```python
from build123d import *

# Parameters (mm, degrees)
BASPROSKE_W         = 6
BASPROSKE_H         = 15
TOOTHCUT_DEPTH      = 23.045407685
TEETHCUTS_COUNT     = 18
TEETHCUTS_ANGLE     = 340
BORSKE_R            = 1.5
BORE_DEPTH          = 50.0000508
EXTRUDE_2_DEPTH     = 6
SKETCH_2_R          = 1.65
CUT_EXTRUDE_1_DEPTH = 6
SKETCH_3_R          = 10.25
CUT_EXTRUDE_2_DEPTH = 2


with BuildPart() as part:
    # BasProSke → Base-Revolve (revolve)
    with BuildSketch(Plane(origin=(0, 0, 0), x_dir=(1, 0, 0), z_dir=(0, 1, 0)), mode=Mode.PRIVATE) as base_revolve_sk:
        with Locations((3, 7.5)):
            Rectangle(BASPROSKE_W, BASPROSKE_H)
    revolve(base_revolve_sk.sketch.rotate(Axis((-10, 0, 0), (1, 0, 0)), 180), axis=Axis((-10, 0, 0), (1, 0, 0)))

    # TooCutSke → ToothCut (cut, through all)
    with BuildSketch(Plane(origin=(0, 0, 0), x_dir=(0, 0, -1), z_dir=(1, 0, 0))):
        with BuildLine():
            ThreePointArc((0.759974923, 11.599129886), (0, 11.624), (-0.759974923, 11.599129886))
            ThreePointArc((-0.759974923, 11.599129886), (-1.229186471, 13.354767823), (-2.254227748, 14.855339189))
            ThreePointArc((-2.254227748, 14.855339189), (0, 15.0254), (2.254227748, 14.855339189))
            ThreePointArc((2.254227748, 14.855339189), (1.229186471, 13.354767823), (0.759974923, 11.599129886))
        make_face()
    toothcut = extrude(amount=TOOTHCUT_DEPTH, mode=Mode.SUBTRACT)

    # TeethCuts: ToothCut ×18 about axis
    teethcuts_axis = Axis((-10, 0, 0), (1, 0, 0))
    for i in range(1, TEETHCUTS_COUNT):
        add(toothcut.rotate(teethcuts_axis, i * TEETHCUTS_ANGLE / (TEETHCUTS_COUNT - 1)), mode=Mode.SUBTRACT)

    # BorSke → Bore (cut, symmetric)
    with BuildSketch(Plane(origin=(0, 0, 0), x_dir=(0, 0, -1), z_dir=(1, 0, 0))):
        with Locations(Location((0, 0, 0), (0, 0, 180))):
            Circle(BORSKE_R)
    extrude(amount=BORE_DEPTH, both=True, mode=Mode.SUBTRACT)

    # Sketch 1 → Extrude 2 (add)
    with BuildSketch(Plane(origin=(6, 0, 0), x_dir=(0, 0, -1), z_dir=(1, 0, 0))):
        Polygon((-10.545854675, -4.889000426), (-42.365659829, -36.708805579), (-42.365659829, -86.708805579), (18.256118436, -121.708805579), (18.256118436, -112.471201272), (-34.365659829, -82.090003426), (-34.365659829, -40.022514078), (-4.889000426, -10.545854675), align=None)
    extrude(amount=-EXTRUDE_2_DEPTH)

    # Sketch 2 → Cut-Extrude 1 (cut)
    with BuildSketch(Plane(origin=(6, 0, 0), x_dir=(0, 0, -1), z_dir=(1, 0, 0))):
        with Locations((-7, 0)):
            Circle(SKETCH_2_R)
        with Locations((0, 7)):
            Circle(SKETCH_2_R)
        with Locations((7, 0)):
            Circle(SKETCH_2_R)
        with Locations((0, -7)):
            Circle(SKETCH_2_R)
    extrude(amount=-CUT_EXTRUDE_1_DEPTH, mode=Mode.SUBTRACT)

    # Sketch 3 → Cut-Extrude 2 (cut)
    with BuildSketch(Plane(origin=(6, 0, 0), x_dir=(0, 0, -1), z_dir=(1, 0, 0))):
        Circle(SKETCH_3_R)
    extrude(amount=-CUT_EXTRUDE_2_DEPTH, mode=Mode.SUBTRACT)


solid = part.part
```
Source: CAD feature listing. Evaluate the final solid. Frame: model axes, mm. A direction names the side the tool comes from. Round coordinates to 2 decimals unless told otherwise and drop trailing zeros. Write each loop counter-clockwise with the first axis right and the second up, starting at its lowest first coordinate (ties: lowest second). Pieces come first, ordered by that corner, then holes. Notation, with made-up numbers: M 51,-5.5 L 85,-5.5 A26 ccw 85,19.5 Z; hole C 74.25,29.25 d7. An arc over 180 degrees is marked long. Answer as a JSON object with one key per item and string values. Group by question number.
(1) Section query D-D on z = 38.5. Output: boundary loops of the cut face in (x, y).
(2) Section query C-C on y = -68. Output: boundary loops of the cut face in (x, z), then the cut area to 3 significant figures.
(3) Section query B-B on x = 1.05. State how many separate pieces and enclosed holes the cut face has, then the cut area to 3 significant figures.
(4) First-contact query: pin 1 (1 mm diameter, centred on x = 1, z = 6, fed in from +Y); pin 2 (10 mm diameter, centred on y = 0, z = 5, fed in from +X); pin 3 (3 mm diameter, centred on y = 0, z = 7, fed in from -X); pin 4 (5 mm diameter, centred on y = 0, z = 0, fed in from -X). Flat tips, straight axial feed; report the tip coordinate or a pass-through.
(5) Section query A-A on z = 19.5. Output: boundary loops of the cut face in (x, y), then the cut area to 3 significant figures.
(6) Reachability of faces 4 (the cylindrical face through (2.96, 10.98, -7.63)), 5 (the cylindrical face through (2.958, 3.506, -12.905)), 6 (the cylindrical face through (2.958, 3.535, 12.946)) from +Z, -Z, +X, -X, +Y, -Y: full face, straight path, thin tool, end or side. Return the list, or none.
(7) Mould query, pull axis Z, two halves, no side actions, for faces 1 (the cylindrical face through (2.958, -3.535, -12.946)), 2 (the cylindrical face through (2.03, 0.07, 8.65)), 3 (the flat face through (6, -53, 35)). Classes: +Z half, -Z half, draft (parallel to the pull), parting line (faces both ways), or undercut.
(8) Ray query, line 1 (Y direction, x = 0.45, z = -8); line 2 (Y direction, x = 2.95, z = 7); line 3 (Y direction, x = 2.9, z = 0). Return the intervals inside material, ascending. Write a range as [from, to].
Computed values:
{
 "1": {"outline": "M 0,-88.94 L 6,-88.94 L 6,-32.84 L 0,-32.84 Z"},
 "2": {"outline": "M 0,34.37 L 6,34.37 L 6,42.37 L 0,42.37 Z", "area": "48.0 mm^2"},
 "3": {"separate pieces": "1", "enclosed holes": "5", "area": "1,730 mm^2"},
 "4": {"pin 1": "y = 12.78", "pin 2": "x = 4", "pin 3": "through", "pin 4": "x = 0"},
 "5": {"outline": "M 0,-99.91 L 6,-99.91 L 6,-90.67 L 0,-90.67 Z; M 0,-25.16 L 6,-25.16 L 6,-13.84 L 0,-13.84 Z", "area": "123 mm^2"},
 "6": {"face 4": "+X, -X", "face 5": "-Z, +X, -X", "face 6": "+Z, +X, -X"},
 "7": {"face 1": "-Z half", "face 2": "undercut", "face 3": "draft"},
 "8": {"line 1": "[-115.79, -106.55], [-8.43, -1.31], [1.31, 8.43]", "line 2": "[-107.13, -97.89], [-13.09, -1.65], [1.65, 9.28], [9.56, 13.09]", "line 3": "[-111.17, -101.93], [-11.62, -8.65], [-5.35, -1.5], [1.5, 5.35], [8.65, 11.62]"}
}
